from build123d import *

# Parameters (mm, degrees)
F0_W      = 850.9
F0_H      = 25.4
F1_DEPTH  = 5.08
F3_DEPTH  = 5.08
F5_DEPTH  = 5.08
F7_DEPTH  = 5.08
F8_W      = 50.8
F8_H      = 749.3
F9_DEPTH  = 5.08
F10_R     = 5.08
F11_W     = 76.2
F11_H     = 50.8
F12_DEPTH = 5.08


with BuildPart() as f1:
    # F0 (on Front) → F1 (new body)
    with BuildSketch(Plane.XZ):
        Polygon((50.8, 50.8), (0, 0), (50.8, 0), (50.8, 25.4), align=None)
        Polygon((0, 749.3), (0, 0), (50.8, 50.8), (50.8, 698.5), align=None)
        Polygon((50.8, 749.3), (0, 749.3), (50.8, 698.5), (50.8, 723.9), align=None)
        with Locations((476.25, 12.7)):
            Rectangle(F0_W, F0_H)
        with Locations((476.25, 736.6)):
            Rectangle(F0_W, F0_H)
        Polygon((901.7, 25.4), (901.7, 0), (952.5, 0), (901.7, 50.8), align=None)
        Polygon((952.5, 749.3), (901.7, 749.3), (901.7, 723.9), (901.7, 698.5), align=None)
        Polygon((901.7, 50.8), (952.5, 0), (952.5, 749.3), (901.7, 698.5), align=None)
    extrude(amount=F1_DEPTH)

    # F2 (on face) → F3 (join)
    with BuildSketch(Plane(origin=(0, 0, 0), x_dir=(1, 0, 0), z_dir=(0, 0, -1))):
        Polygon((0, 50.8), (0, 0), (952.5, 0), (952.5, 50.8), (901.7, 50.8), (901.7, 25.4), (50.8, 25.4), (50.8, 50.8), align=None)
    extrude(amount=-F3_DEPTH)

    # F4 (on face) → F5 (join)
    with BuildSketch(Plane.XY.offset(749.3)):
        Polygon((952.5, 0), (0, 0), (0, -50.8), (50.8, -50.8), (50.8, -25.4), (901.7, -25.4), (901.7, -50.8), (952.5, -50.8), align=None)
    extrude(amount=-F5_DEPTH)

    # F6 (on face) → F7 (join)
    with BuildSketch(Plane(origin=(0, 0, 0), x_dir=(0, -1, 0), z_dir=(-1, 0, 0))):
        Polygon((0.254638, 744.22), (0.254638, 0), (50.8, 0), (50.8, 749.3), align=None)
    extrude(amount=-F7_DEPTH)

    # F8 (on face) → F9 (join)
    with BuildSketch(Plane.YZ.offset(952.5)):
        with Locations((-25.4, 374.65)):
            Rectangle(F8_W, F8_H)
    extrude(amount=-F9_DEPTH)

    # F10
    f10_edges = [f1.edges().sort_by_distance(p)[0] for p in [
        (0, -25.4, 0),
        (5.08, -27.94, 5.08),
        (5.08, -27.94, 744.22),
        (0, -25.4, 749.3),
        (952.5, -25.4, 749.3),
        (947.42, -27.94, 744.22),
        (952.5, -25.4, 0),
        (947.42, -27.94, 5.08),
    ]]
    fillet(f10_edges, radius=F10_R)

    # F11 (on face) → F12 (join)
    with BuildSketch(Plane.XZ.offset(5.08)):
        with Locations((863.6, 698.5)):
            Rectangle(F11_W, F11_H)
        with Locations((863.6, 50.8)):
            Rectangle(F11_W, F11_H)
        with Locations((88.9, 50.8)):
            Rectangle(F11_W, F11_H)
        with Locations((88.9, 698.5)):
            Rectangle(F11_W, F11_H)
    extrude(amount=-F12_DEPTH)


solid = f1.part
Could you check a few things on this model? Use its own coordinates, in mm. A direction names the side the tool comes from. Round coordinates to 2 decimals unless told otherwise and drop trailing zeros. Write each loop counter-clockwise with the first axis right and the second up, starting at its lowest first coordinate (ties: lowest second). Pieces come first, ordered by that corner, then holes. Notation, with made-up numbers: (79.5, 21.25) - (92.5, 21.25) arc R26 cw to (92.5, 54.25) - close; hole circle Ø9 at (12, -33). An arc over 180 degrees is marked (long way). Use a Markdown table: item, result.
Q1. Please list where these lines run through material, in increasing order: L1, parallel to Z at x = 341, y = -10; L2, parallel to X at y = -20, z = 385; L3, parallel to Z at x = 505.5, y = -3.
Output values:
| item | result |
|---|---|
| L1 | 0 to 5.08, 744.22 to 749.3 |
| L2 | 0 to 5.08, 947.42 to 952.5 |
| L3 | 0 to 25.4, 723.9 to 749.3 |
Q2. For pin 1 (13.5 mm diameter, centred on x = 441, y = -38.5, fed in from -Z); pin 2 (4 mm diameter, centred on y = -35, z = 747.5, fed in from -X); pin 3 (5.5 mm diameter, centred on x = 547, z = 3, fed in from -Y); pin 4 (1.5 mm diameter, centred on y = -43, z = 1.5, fed in from -X), each with a flat end and sliding along its axis, tell me the tip position at first contact or that it passes through.
Output values:
| item | result |
|---|---|
| pin 1 | through |
| pin 2 | x = 0.16 |
| pin 3 | y = -25.4 |
| pin 4 | x = 0.86 |
Q3. Thinking about a two-plate mould opening in Z: for faces 1 (the flat face through (474, -5.08, 732)), 2 (the flat face through (483, -14, 749.3)), 3 (the flat face through (403, 0, 737)), which applies, released by +Z, released by -Z, zero draft, split by the parting line, or undercut?
Output values:
| item | result |
|---|---|
| face 1 | undercut |
| face 2 | released by +Z |
| face 3 | zero draft |
Q4. For faces 4 (the flat face through (470, -18, 5.08)), 5 (the flat face through (470, -14, 0)), which set-ups out of +Z, -Z, +X, -X, +Y, -Y let a thin tool reach every point of the face, with its end or its side?
Output values:
| item | result |
|---|---|
| face 4 | -Y |
| face 5 | -Z, +X, -X, +Y, -Y |
Q5. I want a section at A-A (y = -43). List the corners of the cut face in (x, z) for me, plus the area to 3 significant figures.
Output values:
| item | result |
|---|---|
| outline | (0, 5.08) arc R5.08 ccw to (5.08, 0) - (50.8, 0) - (50.8, 5.08) - (10.16, 5.08) arc R5.08 cw to (5.08, 10.16) - (5.08, 739.14) arc R5.08 cw to (10.16, 744.22) - (50.8, 744.22) - (50.8, 749.3) - (5.08, 749.3) arc R5.08 ccw to (0, 744.22) - close; (901.7, 0) - (947.42, 0) arc R5.08 ccw to (952.5, 5.08) - (952.5, 744.22) arc R5.08 ccw to (947.42, 749.3) - (901.7, 749.3) - (901.7, 744.22) - (942.34, 744.22) arc R5.08 cw to (947.42, 739.14) - (947.42, 10.16) arc R5.08 cw to (942.34, 5.08) - (901.7, 5.08) - close |
| area | 8,540 mm2 |
Q6. I want a section at B-B (x = 862). List the corners of the cut face in (y, z) for me, plus the area to 3 significant figures.
Output values:
| item | result |
|---|---|
| outline | (-25.4, 0) - (0, 0) - (0, 76.2) - (-5.08, 76.2) - (-5.08, 5.08) - (-25.4, 5.08) - close; (-25.4, 744.22) - (-5.08, 744.22) - (-5.08, 673.1) - (0, 673.1) - (0, 749.3) - (-25.4, 749.3) - close |
| area | 981 mm2 |
Q7. I want a section at C-C (z = 233.5). List the corners of the cut face in (x, y) for me.
Output values:
| item | result |
|---|---|
| outline | (0, -50.8) - (5.08, -50.8) - (5.08, -5.08) - (50.8, -5.08) - (50.8, 0) - (0, 0) - close; (901.7, -5.08) - (947.42, -5.08) - (947.42, -50.8) - (952.5, -50.8) - (952.5, 0) - (901.7, 0) - close |
